Input: dimensioned drawing with shaded views. Units: mm. Origin: part minimum x, y, z. A direction names the side the tool comes from. Round coordinates to 2 decimals unless told otherwise and drop trailing zeros. Loops run counter-clockwise (first coordinate to the right, second up) from the corner with the lowest first, then second, coordinate; pieces in that order, holes last. Notation, with made-up numbers: M 7.25,41 L 64.25,41 A25 cw 64.25,63 Z; hole C 17,84 d10. An arc over 180 degrees is marked long. Use one line per item in the form item = value. Start each with the question number.
Q1. First-contact query: P1, Ø2, axis at x = 15, z = 11, coming from the -Y side. Flat tip, straight axial feed; report the tip coordinate or a pass-through.
Q2. Access query for the marked faces 1 and 2. Directions: +Z, -Z, +X, -X, +Y, -Y. A direction counts if a zero-diameter tool reaches every point of the face in a straight line with its end or side. Return the directions, or none.
Q3. Section query D-D, the plane y = 13. Output: boundary loops of the cut face in (x, z), and give its area (3 significant figures).
Q4. Mould query, pull axis Z, two halves, no side actions, for the marked faces 3, 4 and 5. Classes: pulls with the +Z half, pulls with the -Z half, needs draft (parallel to the pull), parting line crosses it, or undercut.
Q5. Ray query, line 1 along Z through (x, y) = (10, 34); line 2 along Y through (x, z) = (18.75, 14.5); line 3 along X through (y, z) = (28.5, 13). Return the intervals inside material, ascending.
Q6. Section query A-A, the plane y = 21. Output: boundary loops of the cut face in (x, z).
Q7. Section query C-C, the plane z = 4.5. Output: boundary loops of the cut face in (x, y), and give its area (3 significant figures).
Q8. Section query B-B, the plane x = 5. Output: boundary loops of the cut face in (y, z).
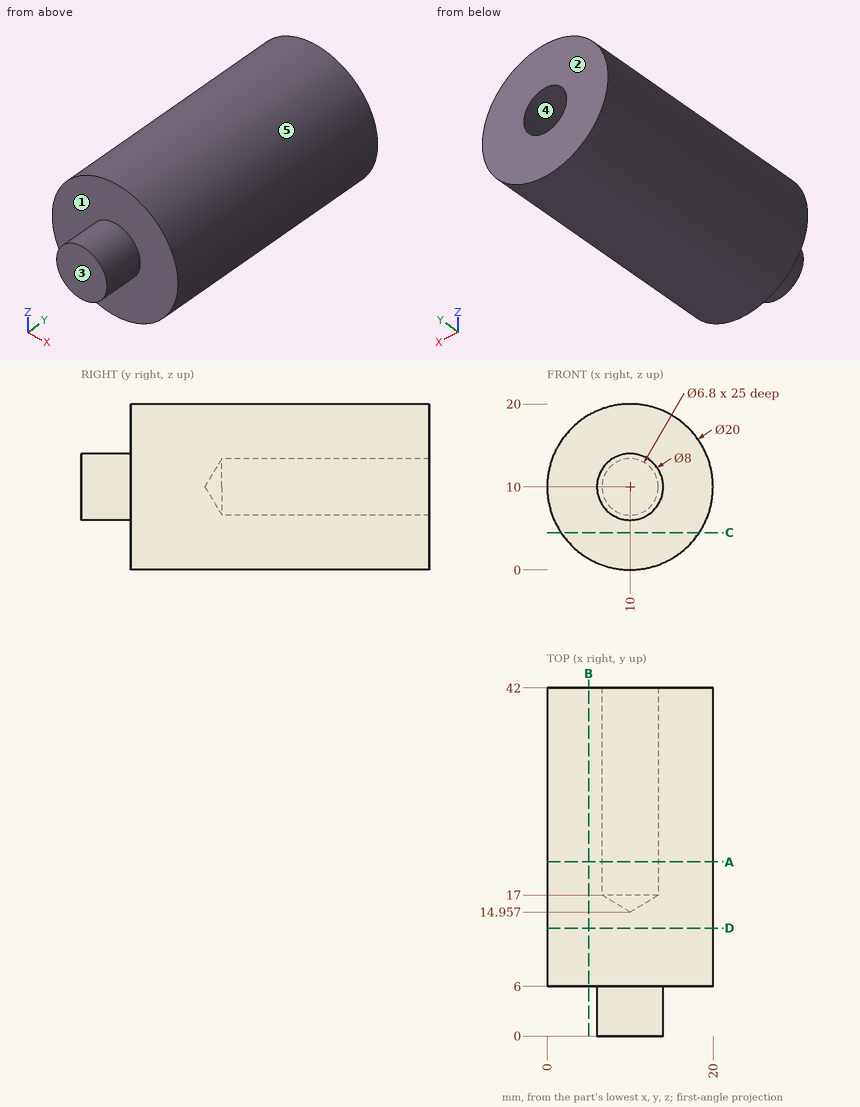
Results found:
q1.P1 = 6
q2.face_1 = -Y
q2.face_2 = +Z, -Z, +X, -X, +Y
q3.outline = C 10,10 d20
q3.area = 314 mm²
q4.face_3 = needs draft
q4.face_4 = undercut
q4.face_5 = parting line crosses it
q5.line_1 = 0 to 6.6, 13.4 to 20
q5.line_2 = 6 to 42
q5.line_3 = 0.46 to 8.4, 11.6 to 19.54
q6.outline = C 10,10 d20; hole C 10,10 d6.8
q7.outline = M 1.65,6 L 18.35,6 L 18.35,42 L 1.65,42 Z
q7.area = 601 mm²
q8.outline = M 6,1.34 L 42,1.34 L 42,18.66 L 6,18.66 Z
